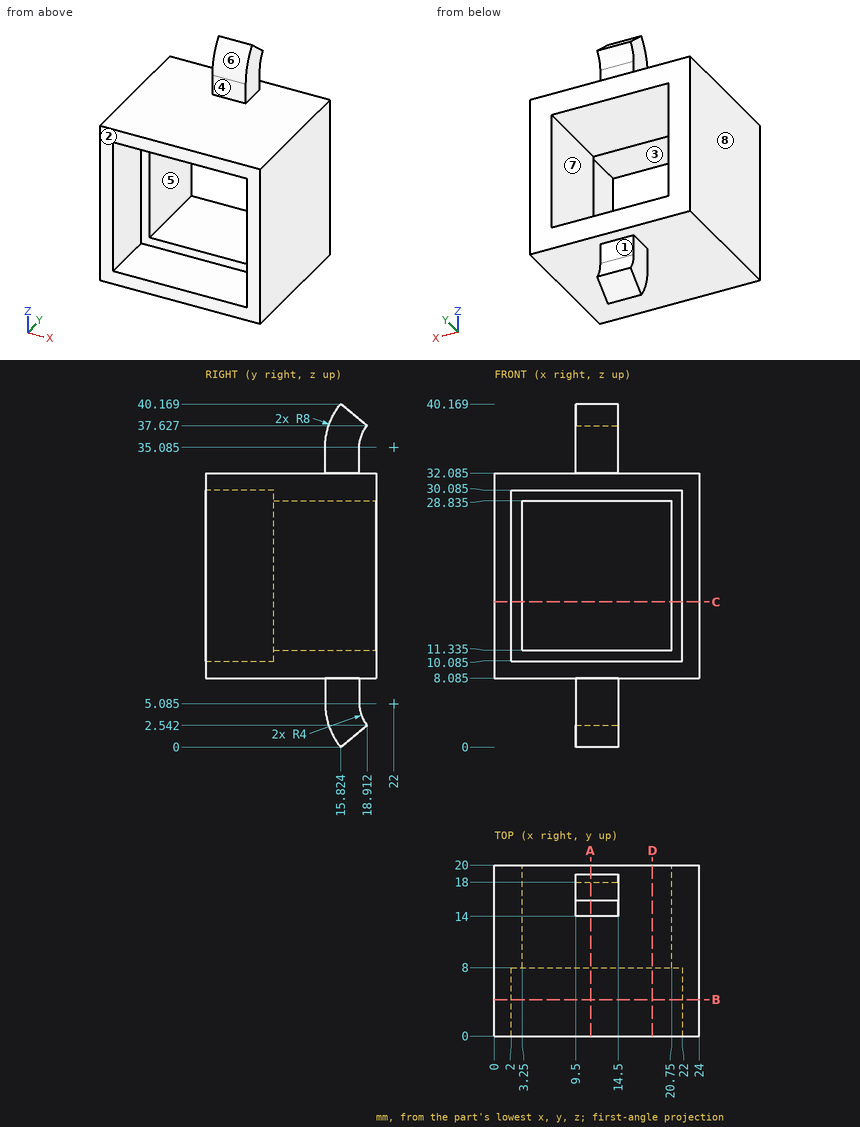
Input: dimensioned drawing with shaded views. Units: mm. Origin: part minimum x, y, z. A direction names the side the tool comes from. Round coordinates to 2 decimals unless told otherwise and drop trailing zeros. Loops run counter-clockwise (first coordinate to the right, second up) from the corner with the lowest first, then second, coordinate; pieces in that order, holes last. Notation, with made-up numbers: (56.5, -20) -> (107.5, -20) arc R24 ccw to (107.5, -3) -> close; hole circle Ø9 at (54.25, -30). An arc over 180 degrees is marked (long way). One line per item, written item: value.
(1) Set-up query: the marked faces 1, 2, 3, 4 and 5. Return all of +Z, -Z, +X, -X, +Y, -Y with unobstructed straight access to the full face (end or side cutting, diameter ignored); none if empty.
Geometry check:
face 1: +X, -X, +Y
face 2: +Z, -Z, +X, -X, -Y
face 3: -Y
face 4: +Z, +X, -X, -Y
face 5: +Y, -Y
(2) Pin query (flat end, axial travel): pin 1 (3.5 mm diameter, centred on x = 13, z = 33, fed in from -Y); pin 2 (1.5 mm diameter, centred on x = 14.5, y = 7, fed in from +Z) (1 decimal); pin 3 (1.5 mm diameter, centred on x = 13, z = 34.5, fed in from +Y); pin 4 (2.5 mm diameter, centred on y = 16, z = 2.5, fed in from +X). Return the tip coordinate at first contact, or that it passes through.
Geometry check:
pin 1: y = 0
pin 2: z = 32.1
pin 3: y = 18
pin 4: x = 14.5
(3) Section B-B (y = 4.25). Return the cut outline in (x, z) (1 decimal), plus the area to 3 significant figures.
Geometry check:
outline: (0, 8.1) -> (24, 8.1) -> (24, 32.1) -> (0, 32.1) -> close; hole (2, 10.1) -> (22, 10.1) -> (22, 30.1) -> (2, 30.1) -> close
area: 176 mm2
(4) Material intervals for line 1 (Z direction, x = 16, y = 14.25) (1 decimal); line 2 (X direction, y = 10.25, z = 22); line 3 (Z direction, x = 13.25, y = 6) (1 decimal), sorted ascending. Write a range as [from, to].
Geometry check:
line 1: [8.1, 11.3], [28.8, 32.1]
line 2: [0, 3.25], [20.75, 24]
line 3: [8.1, 10.1], [30.1, 32.1]
(5) Section A-A (x = 11.25). Return the cut outline in (y, z) (1 decimal), plus the area to 3 significant figures.
Geometry check:
outline: (0, 8.1) -> (14, 8.1) -> (14, 5.1) arc R8 ccw to (15.8, 0) -> (18.9, 2.5) arc R4 cw to (18, 5.1) -> (18, 8.1) -> (20, 8.1) -> (20, 11.3) -> (8, 11.3) -> (8, 10.1) -> (0, 10.1) -> close; (0, 30.1) -> (8, 30.1) -> (8, 28.8) -> (20, 28.8) -> (20, 32.1) -> (18, 32.1) -> (18, 35.1) arc R4 cw to (18.9, 37.6) -> (15.8, 40.2) arc R8 ccw to (14, 35.1) -> (14, 32.1) -> (0, 32.1) -> close
area: 167 mm2
(6) Section D-D (x = 18.5). Return the cut outline in (y, z) (1 decimal), plus the area to 3 significant figures.
Geometry check:
outline: (0, 8.1) -> (20, 8.1) -> (20, 11.3) -> (8, 11.3) -> (8, 10.1) -> (0, 10.1) -> close; (0, 30.1) -> (8, 30.1) -> (8, 28.8) -> (20, 28.8) -> (20, 32.1) -> (0, 32.1) -> close
area: 110 mm2
(7) Mould query, pull axis Z, two halves, no side actions, for the marked faces 6, 7 and 8. Classes: pulls with the +Z half, pulls with the -Z half, needs draft (parallel to the pull), parting line crosses it, or undercut.
Geometry check:
face 6: pulls with the +Z half
face 7: undercut
face 8: needs draft
(8) Section C-C (z = 17). Return the cut outline in (x, y), plus the area to 3 significant figures.
Geometry check:
outline: (0, 0) -> (2, 0) -> (2, 8) -> (3.25, 8) -> (3.25, 20) -> (0, 20) -> close; (20.75, 8) -> (22, 8) -> (22, 0) -> (24, 0) -> (24, 20) -> (20.75, 20) -> close
area: 110 mm2
